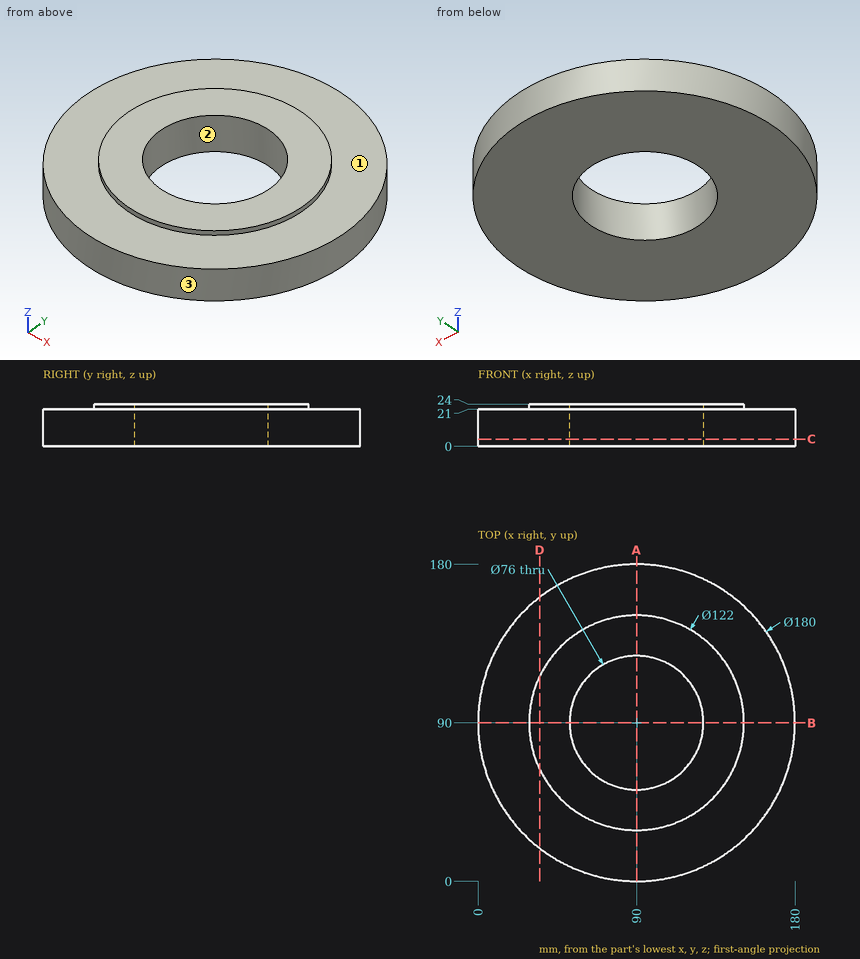
Here's the drawing with two shaded views (mm, measured from the low corner). I have some questions. Round coordinates to 2 decimals unless told otherwise and drop trailing zeros. Loops run counter-clockwise (first coordinate to the right, second up) from the corner with the lowest first, then second, coordinate; pieces in that order, holes last.
Item 1: Suppose I cut it at D-D, the plane x = 35. Write out the boundary of the cut face in (y, z).
Item 2: If we mould it in two halves opening along X, with no side actions, what happens to the marked faces 1, 2 and 3? For each: +X half, -X half, draft (parallel to the pull), parting line (faces both ways), or undercut.
Item 3: Suppose I cut it at A-A, the plane x = 90. Write out the boundary of the cut face in (y, z).
Item 4: Suppose I cut it at C-C, the plane z = 4. Write out the boundary of the cut face in (x, y), then the cut area to 3 significant figures.
Item 5: Please list where these lines run through material, in increasing order: L1, parallel to Y at x = 90, z = 6; L2, parallel to Z at x = 127.5, y = 37; L3, parallel to Y at x = 71, z = 22.5.
Item 6: Will these pins go through, and if not, where does the flat tip stop? pin 1 Ø4 at (x, z) = (32, 13) entering from +Y; pin 2 Ø4 at (x, z) = (22.5, 18.5) entering from -Y; pin 3 Ø6 at (y, z) = (149.5, 4.5) entering from +X.
Reported:
1. outline: (18.76, 0) - (161.24, 0) - (161.24, 21) - (116.38, 21) - (116.38, 24) - (63.62, 24) - (63.62, 21) - (18.76, 21) - close
2. face 1: draft
2. face 2: undercut
2. face 3: parting line
3. outline: (0, 0) - (52, 0) - (52, 24) - (29, 24) - (29, 21) - (0, 21) - close; (128, 0) - (180, 0) - (180, 21) - (151, 21) - (151, 24) - (128, 24) - close
4. outline: circle Ø180 at (90, 90); hole circle Ø76 at (90, 90)
4. area: 20,900 mm2
5. L1: y = 0 to 52, 128 to 180
5. L2: z = 0 to 21
5. L3: y = 32.03 to 57.09, 122.91 to 147.97
6. pin 1: stops at y = 160.46
6. pin 2: stops at y = 28.28
6. pin 3: stops at x = 160.06
